Can you work these out from the model? Positions are in its coordinate system, mm. A direction names the side the tool comes from. Coordinates: 2 decimals unless noted, no trailing zeros. Loops run counter-clockwise (first coordinate to the right, second up) from the corner with the lowest first, then second, coordinate; pieces in that order, holes last.
```python
from build123d import *

# Parameters (mm, degrees)
SKETCH3_R           = 5.2578
BOSS_EXTRUDE1_DEPTH = 0.76708
BOSS_EXTRUDE2_DEPTH = 3.06832
BOSS_EXTRUDE2_TAPER = 1
SKETCH5_OUTSIDE_W   = 62.562
SKETCH5_OUTSIDE_H   = 62.562
SKETCH5_OUTSIDE_R   = 3.7703125
CUT_EXTRUDE1_DEPTH  = 19.130316457
CUT_EXTRUDE1_DRAFT  = -50
SKETCH6_R           = 3.39328125
CUT_EXTRUDE2_DEPTH  = 0.38354
CUT_EXTRUDE2_DRAFT  = -45
CUT_EXTRUDE3_START  = 3.8354
SKETCH10_W          = 8.334375
SKETCH10_H          = 0.9921875
CUT_EXTRUDE3_DEPTH  = 0.76708


with BuildPart() as part:
    # Sketch2 → Revolve1 (revolve)
    with BuildSketch(Plane(origin=(0, 0, 0), x_dir=(0, 0, -1), z_dir=(1, 0, 0))):
        Polygon((0, 0), (0, 2.413), (11.959166667, 2.413), (12.7, 1.672166667), (12.7, 0), align=None)
    revolve(axis=Axis((0, 0, -12.7), (0, 0, 1)))

    # Sketch3 → Boss-Extrude1 (add)
    with BuildSketch(Plane.XY):
        Circle(SKETCH3_R)
    extrude(amount=BOSS_EXTRUDE1_DEPTH)

    # Sketch4 → Boss-Extrude2 (add)
    with BuildSketch(Plane.XY.offset(0.76708)):
        Polygon((-3.96875, 2.291358881), (-3.96875, -2.291358881), (0, -4.582717762), (3.96875, -2.291358881), (3.96875, 2.291358881), (0, 4.582717762), align=None)
    extrude(amount=BOSS_EXTRUDE2_DEPTH, taper=BOSS_EXTRUDE2_TAPER)


with BuildPart() as cut_extrude1_tool:
    # Sketch5 outside → Cut-Extrude1 (with draft: the straight prism first)
    with BuildSketch(Plane.XY.offset(3.8354)):
        Rectangle(SKETCH5_OUTSIDE_W, SKETCH5_OUTSIDE_H)
        Circle(SKETCH5_OUTSIDE_R, mode=Mode.SUBTRACT)
    extrude(amount=-CUT_EXTRUDE1_DEPTH)
    # Cut-Extrude1: the draft: its side faces are tilted about the plane it starts from
    cut_extrude1_sides = [cut_extrude1_tool.faces().sort_by_distance(p)[0] for p in [
        (0, -31.281, -5.729758229),
        (31.281, 0, -5.729758229),
        (0, 31.281, -5.729758229),
        (-31.281, 0, -5.729758229),
        (-3.7703125, 0, -5.729758229),
    ]]
    draft(cut_extrude1_sides, Plane.XY.offset(3.8354), CUT_EXTRUDE1_DRAFT)


with BuildPart() as part_1:
    add(part.part)

    # Cut-Extrude1: cut by cut_extrude1_tool
    add(cut_extrude1_tool.part, mode=Mode.SUBTRACT)


with BuildPart() as cut_extrude2_tool:
    # Sketch6 → Cut-Extrude2 (with draft: the straight prism first)
    with BuildSketch(Plane.XY.offset(3.8354)):
        Circle(SKETCH6_R)
    extrude(amount=-CUT_EXTRUDE2_DEPTH)
    # Cut-Extrude2: the draft: its side faces are tilted about the plane it starts from
    cut_extrude2_sides = [cut_extrude2_tool.faces().sort_by_distance(p)[0] for p in [
        (-3.39328125, 0, 3.64363),
    ]]
    draft(cut_extrude2_sides, Plane.XY.offset(3.8354), CUT_EXTRUDE2_DRAFT)


with BuildPart() as part_2:
    add(part_1.part)

    # Cut-Extrude2: cut by cut_extrude2_tool
    add(cut_extrude2_tool.part, mode=Mode.SUBTRACT)

    # Sketch10 → Cut-Extrude3 (cut)
    with BuildSketch(Plane.XY.offset(CUT_EXTRUDE3_START)):
        Rectangle(SKETCH10_W, SKETCH10_H)
    extrude(amount=-CUT_EXTRUDE3_DEPTH, mode=Mode.SUBTRACT)


solid = part_2.part
```
(1) I want a section at A-A on y = 0. Write out the boundary of the cut face in (x, z).
Check values:
outline: (-5.26, 0) - (-2.41, 0) - (-2.41, -11.96) - (-1.67, -12.7) - (1.67, -12.7) - (2.41, -11.96) - (2.41, 0) - (5.26, 0) - (5.26, 0.77) - (3.97, 0.77) - (3.93, 3.07) - (-3.93, 3.07) - (-3.97, 0.77) - (-5.26, 0.77) - close
(2) If we mould it in two halves opening along X, with no side actions, what happens to faces 4 (the flat face through (2.3, 1.2, 0)), 5 (the conical face through (0.079, 3.891, 3.733)), 6 (the conical face through (-0.06, -3.12, 3.56))? For each: released by +X, released by -X, zero draft, split by the parting line, or undercut.
Check values:
face 4: zero draft
face 5: split by the parting line
face 6: undercut
(3) If I drill on probe 1 along Z at (x, y) = (4, -2.5); probe 2 along X at (y, z) = (0.5, 3); probe 3 along Z at (x, y) = (-2.75, -0.75), over which ranges is the centre line in solid material (lowest first)?
Check values:
probe 1: z = 0 to 0.77
probe 2: x = -3.93 to 3.93
probe 3: z = 0 to 3.45
(4) I want a section at C-C on z = -6.25. Write out the boundary of the cut face in (x, y), then the cut area to 3 significant figures.
Check values:
outline: circle Ø4.83 at (0, 0)
area: 18.3 mm2
(5) I want a section at B-B on z = 2.75. Write out the boundary of the cut face in (x, y), then the cut area to 3 significant figures.
Check values:
outline: (-3.93, -2.27) - (0, -4.54) - (3.93, -2.27) - (3.93, 2.27) - (0, 4.54) - (-3.93, 2.27) - close
area: 53.6 mm2
(6) I'm going to push flat-ended pins straight in: pin 1 (5 mm diameter, centred on x = 1.5, z = -5, fed in from +Y); pin 2 (0.8 mm diameter, centred on x = -1.5, z = 3.5, fed in from +Y); pin 3 (3 mm diameter, centred on x = 0.5, y = -1.5, fed in from +Z); pin 4 (1.5 mm diameter, centred on y = -4, z = -10.5, fed in from -X). Where does each tip first touch, or does it pass through?
Check values:
pin 1: stops at y = 2.41
pin 2: stops at y = 3.89
pin 3: stops at z = 3.52
pin 4: passes through
(7) Which directions (+Z, -Z, +X, -X, +Y, -Y) give clear straight access to the entire face, cutting with the end or side of a thin tool? Please do faces 1 (the conical face through (-0.079, -3.891, 3.733)), 2 (the cylindrical face through (1.468, -1.915, -6.063)), 3 (the flat face through (2, -4, 0.767)).
Check values:
face 1: +Z, -Y
face 2: -Z
face 3: +Z
